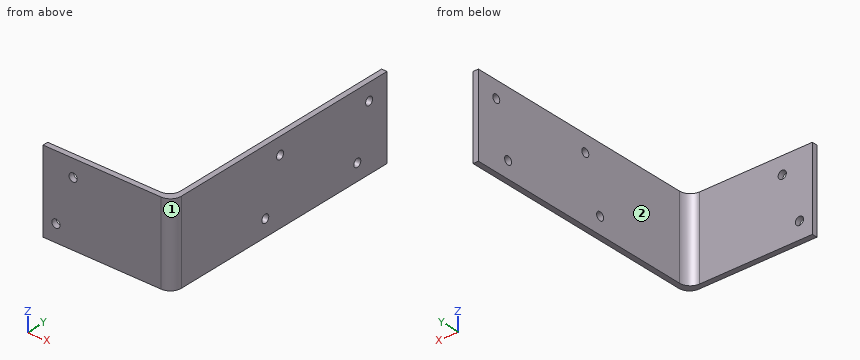
from build123d import *

# Parameters (mm, degrees)
BOSS_EXTRUDE1_DEPTH = 38.4429
SKETCH2_R           = 1.9177
CUT_EXTRUDE1_DEPTH  = 3.54
SKETCH3_R           = 1.9177
CUT_EXTRUDE2_DEPTH  = 3.54
FILLET1_R           = 5.08
SKETCH4_W           = 52.9336
SKETCH4_H           = 38.4429
CUT_EXTRUDE4_DEPTH  = 3.54


with BuildPart() as part:
    # Sketch1 → Boss-Extrude1 (new body)
    with BuildSketch(Plane.XY):
        Polygon((0, 0), (113.4872, 0), (113.4872, 118.4148), (110.9472, 118.4148), (110.9472, 2.54), (0, 2.54), align=None)
    extrude(amount=BOSS_EXTRUDE1_DEPTH)

    # Sketch2 → Cut-Extrude1 (cut, through all)
    with BuildSketch(Plane(origin=(0, 2.54, 0), x_dir=(1, 0, 0), z_dir=(0, 1, 0))):
        with Locations((67.0687, -30.4292)):
            Circle(SKETCH2_R)
        with Locations((59.0042, -8.0137)):
            Circle(SKETCH2_R)
        with Locations((16.2052, -30.4292)):
            Circle(SKETCH2_R)
        with Locations((9.8806, -8.0137)):
            Circle(SKETCH2_R)
    extrude(amount=-CUT_EXTRUDE1_DEPTH, mode=Mode.SUBTRACT)

    # Sketch3 → Cut-Extrude2 (cut, through all)
    with BuildSketch(Plane.ZY.offset(-110.9472)):
        with Locations((7.8232, 51.3842)):
            Circle(SKETCH3_R)
        with Locations((30.6197, 59.5249)):
            Circle(SKETCH3_R)
        with Locations((7.8232, 102.0699)):
            Circle(SKETCH3_R)
        with Locations((30.6197, 108.5723)):
            Circle(SKETCH3_R)
    extrude(amount=-CUT_EXTRUDE2_DEPTH, mode=Mode.SUBTRACT)

    # Fillet1
    fillet1_edges = [part.edges().sort_by_distance(p)[0] for p in [
        (110.9472, 2.54, 19.22145),
        (113.4872, 0, 19.22145),
    ]]
    fillet(fillet1_edges, radius=FILLET1_R)

    # Sketch4 → Cut-Extrude4 (cut, through all)
    with BuildSketch(Plane(origin=(0, 2.54, 0), x_dir=(1, 0, 0), z_dir=(0, 1, 0))):
        with Locations((26.4668, -19.22145)):
            Rectangle(SKETCH4_W, SKETCH4_H)
    extrude(amount=-CUT_EXTRUDE4_DEPTH, mode=Mode.SUBTRACT)


solid = part.part
Work out the finished part from the listing and answer in its coordinate system (mm). Face numbers are marked on the shaded views. A direction names the side the tool comes from. Coordinates: 2 decimals unless noted, no trailing zeros. Write each loop counter-clockwise with the first axis right and the second up, starting at its lowest first coordinate (ties: lowest second). Pieces come first, ordered by that corner, then holes. Notation, with made-up numbers: M 60,34 L 97,34 A11 ccw 97,50 Z; hole C 81.5,25.5 d1. An arc over 180 degrees is marked long. Use one line per item in the form item = value. Start each with the question number.
1. Each of these flat-tipped pins is pushed along its axis until it touches: P1, Ø19, axis at x = 68, z = 18.5, coming from the +Y side; P2, Ø2.5, axis at y = 59.52, z = 30.62, coming from the -X side; P3, Ø19, axis at y = 66, z = 25, coming from the -X side. Where does it stop, or does it pass through?
2. A tool of negligible diameter and unlimited length cuts with its end or side. For the marked faces 1 and 2, from which of +Z, -Z, +X, -X, +Y, -Y can it reach the whole face along a straight path? Write none if from no direction.
3. The part is cut by section A-A (z = 34). Give the vertices of the cut face in (x, y), plus the area to 3 significant figures.
4. The part is cut by section C-C (x = 98.5). Give the vertices of the cut face in (y, z), plus the area to 3 significant figures.
5. The part is cut by section B-B (y = 18.5). Give the vertices of the cut face in (x, z), plus the area to 3 significant figures.
6. Straight lines are drawn through the part: probe 1 along X at (y, z) = (81, 4); probe 2 along Y at (x, z) = (69.5, 3). For each, find the intervals that lie inside material, in ascending order. Write a range as from..to.
Evaluation:
q1.P1 = 2.54
q1.P2 = through
q1.P3 = 110.95
q2.face_1 = +Z, -Z, +X, -Y
q2.face_2 = +Z, -Z, -X, +Y
q3.outline = M 52.93,0 L 108.41,0 A5.08 ccw 113.49,5.08 L 113.49,118.41 L 110.95,118.41 L 110.95,7.62 A5.08 cw 105.87,2.54 L 52.93,2.54 Z
q3.area = 448 mm^2
q4.outline = M 0,0 L 2.54,0 L 2.54,38.44 L 0,38.44 Z
q4.area = 97.6 mm^2
q5.outline = M 110.95,0 L 113.49,0 L 113.49,38.44 L 110.95,38.44 Z
q5.area = 97.6 mm^2
q6.probe_1 = 110.95..113.49
q6.probe_2 = 0..2.54
